For this review, take the finished solid that the model builds, in its own axes (mm). A direction names the side the tool comes from. Give positions to 0.01 mm unless a question says otherwise; leave off trailing zeros. Write each loop counter-clockwise with the first axis right and the second up, starting at its lowest first coordinate (ties: lowest second). Pieces come first, ordered by that corner, then holes. Notation, with made-up numbers: M 40,69 L 68,69 A13 ccw 68,82 Z; hole C 66,55 d5. An arc over 180 degrees is marked long. Use one line per item in the form item = value. Start each with the question number.
Q1. Consider section C-C on z = 25. Write out the cut boundary in (x, y), and give its area (3 significant figures).
Q2. Mouldability with a two-part tool opening along X and no side actions: class faces 3 (the flat face through (25, 202, 50)), 4 (the flat face through (25, 200, 2.5)), 5 (the flat face through (0, 197, 25)) as released by +X, released by -X, zero draft, split by the parting line, or undercut.
Q3. Consider section B-B on x = 18. Write out the cut boundary in (y, z), and give its area (3 significant figures).
Q4. For probe 1 along Z at (x, y) = (38.5, 160); probe 2 along X at (y, z) = (382.5, 3), list the stretches that pass through material, from the lowest coordinate up. Write a range as [from, to].
Q5. Tool access review of faces 1 (the flat face through (25, 0, 1)), 2 (the flat face through (47.5, 200, 25)): name each direction out of +Z, -Z, +X, -X, +Y, -Y from which nothing blocks a thin tool from reaching the whole face with its end or side.
Q6. Consider section A-A on y = 349. Write out the cut boundary in (x, z), and give its area (3 significant figures).
```python
from build123d import *

# Parameters (mm, degrees)
SKETCH1_W           = 50
SKETCH1_H           = 400
BOSS_EXTRUDE1_DEPTH = 50
SKETCH2_W           = 45
SKETCH2_H           = 45
CUT_EXTRUDE1_DEPTH  = 407.201920232
FILLET1_R           = 5
FILLET2_R           = 5


with BuildPart() as part:
    # Sketch1 → Boss-Extrude1 (new body)
    with BuildSketch(Plane.XY):
        with Locations((25, 200)):
            Rectangle(SKETCH1_W, SKETCH1_H)
    extrude(amount=BOSS_EXTRUDE1_DEPTH)

    # Sketch2 → Cut-Extrude1 (cut, through all)
    with BuildSketch(Plane(origin=(0, 400, 0), x_dir=(1, 0, 0), z_dir=(0, 1, 0))):
        with Locations((25, -25)):
            Rectangle(SKETCH2_W, SKETCH2_H)
    extrude(amount=-CUT_EXTRUDE1_DEPTH, mode=Mode.SUBTRACT)

    # Fillet1
    fillet1_edges = [part.edges().sort_by_distance(p)[0] for p in [
        (50, 200, 50),
        (0, 200, 50),
        (50, 200, 0),
        (0, 200, 0),
    ]]
    fillet(fillet1_edges, radius=FILLET1_R)

    # Fillet2
    # the kernel refuses this fillet: 5 mm, written as the material it takes off along each edge
    with BuildSketch(Plane(origin=(47.5, 400, 2.5), x_dir=(0, -1, 0), z_dir=(0, 0, 1)), Plane(origin=(47.5, 400, 47.5), x_dir=(0, -1, 0), z_dir=(-1, 0, 0)), Plane(origin=(2.5, 400, 47.5), x_dir=(0, -1, 0), z_dir=(0, 0, -1)), Plane(origin=(2.5, 400, 2.5), x_dir=(0, -1, 0), z_dir=(1, 0, 0))) as fillet2_piece_1:
        with BuildLine():
            CenterArc((FILLET2_R, FILLET2_R), FILLET2_R, 180, 90)
            Line((0, FILLET2_R), (-FILLET2_R * 0.02, FILLET2_R))
            Line((-FILLET2_R * 0.02, FILLET2_R), (-FILLET2_R * 0.02, -FILLET2_R * 0.02))
            Line((-FILLET2_R * 0.02, -FILLET2_R * 0.02), (FILLET2_R, -FILLET2_R * 0.02))
            Line((FILLET2_R, -FILLET2_R * 0.02), (FILLET2_R, 0))
        make_face()
    extrude(amount=45, mode=Mode.SUBTRACT)
    with BuildSketch(Plane(origin=(47.5, 400, -10), x_dir=(0, -1, 0), z_dir=(0, 0, 1))) as fillet2_piece_2a_section:
        with BuildLine():
            CenterArc((FILLET2_R, FILLET2_R), FILLET2_R, 180, 90)
            Line((0, FILLET2_R), (-FILLET2_R * 0.02, FILLET2_R))
            Line((-FILLET2_R * 0.02, FILLET2_R), (-FILLET2_R * 0.02, -FILLET2_R * 0.02))
            Line((-FILLET2_R * 0.02, -FILLET2_R * 0.02), (FILLET2_R, -FILLET2_R * 0.02))
            Line((FILLET2_R, -FILLET2_R * 0.02), (FILLET2_R, 0))
        make_face()
    fillet2_piece_2a = extrude(amount=57.5, mode=Mode.PRIVATE)
    fillet2_piece_2a = split(fillet2_piece_2a, bisect_by=Plane(origin=(48.631975571, 398.868024429, 2.5), z_dir=(0, 0, -1)), keep=Keep.TOP, mode=Mode.PRIVATE)
    with BuildSketch(Plane(origin=(2.5, 400, 2.5), x_dir=(0, -1, 0), z_dir=(1, 0, 0))) as fillet2_piece_2b_section:
        with BuildLine():
            CenterArc((FILLET2_R, FILLET2_R), FILLET2_R, 180, 90)
            Line((0, FILLET2_R), (-FILLET2_R * 0.02, FILLET2_R))
            Line((-FILLET2_R * 0.02, FILLET2_R), (-FILLET2_R * 0.02, -FILLET2_R * 0.02))
            Line((-FILLET2_R * 0.02, -FILLET2_R * 0.02), (FILLET2_R, -FILLET2_R * 0.02))
            Line((FILLET2_R, -FILLET2_R * 0.02), (FILLET2_R, 0))
        make_face()
    fillet2_piece_2b = extrude(amount=57.5, mode=Mode.PRIVATE)
    fillet2_piece_2b = split(fillet2_piece_2b, bisect_by=Plane(origin=(47.5, 398.868024429, 1.368024429), z_dir=(1, 0, 0)), keep=Keep.TOP, mode=Mode.PRIVATE)
    fillet2_piece_2 = fillet2_piece_2a & fillet2_piece_2b
    add(fillet2_piece_2, mode=Mode.SUBTRACT)
    with BuildSketch(Plane(origin=(60, 400, 47.5), x_dir=(0, -1, 0), z_dir=(-1, 0, 0))) as fillet2_piece_3a_section:
        with BuildLine():
            CenterArc((FILLET2_R, FILLET2_R), FILLET2_R, 180, 90)
            Line((0, FILLET2_R), (-FILLET2_R * 0.02, FILLET2_R))
            Line((-FILLET2_R * 0.02, FILLET2_R), (-FILLET2_R * 0.02, -FILLET2_R * 0.02))
            Line((-FILLET2_R * 0.02, -FILLET2_R * 0.02), (FILLET2_R, -FILLET2_R * 0.02))
            Line((FILLET2_R, -FILLET2_R * 0.02), (FILLET2_R, 0))
        make_face()
    fillet2_piece_3a = extrude(amount=57.5, mode=Mode.PRIVATE)
    fillet2_piece_3a = split(fillet2_piece_3a, bisect_by=Plane(origin=(47.5, 398.868024429, 48.631975571), z_dir=(1, 0, 0)), keep=Keep.TOP, mode=Mode.PRIVATE)
    with BuildSketch(Plane(origin=(47.5, 400, 2.5), x_dir=(0, -1, 0), z_dir=(0, 0, 1))) as fillet2_piece_3b_section:
        with BuildLine():
            CenterArc((FILLET2_R, FILLET2_R), FILLET2_R, 180, 90)
            Line((0, FILLET2_R), (-FILLET2_R * 0.02, FILLET2_R))
            Line((-FILLET2_R * 0.02, FILLET2_R), (-FILLET2_R * 0.02, -FILLET2_R * 0.02))
            Line((-FILLET2_R * 0.02, -FILLET2_R * 0.02), (FILLET2_R, -FILLET2_R * 0.02))
            Line((FILLET2_R, -FILLET2_R * 0.02), (FILLET2_R, 0))
        make_face()
    fillet2_piece_3b = extrude(amount=57.5, mode=Mode.PRIVATE)
    fillet2_piece_3b = split(fillet2_piece_3b, bisect_by=Plane(origin=(48.631975571, 398.868024429, 47.5), z_dir=(0, 0, 1)), keep=Keep.TOP, mode=Mode.PRIVATE)
    fillet2_piece_3 = fillet2_piece_3a & fillet2_piece_3b
    add(fillet2_piece_3, mode=Mode.SUBTRACT)
    with BuildSketch(Plane(origin=(2.5, 400, 60), x_dir=(0, -1, 0), z_dir=(0, 0, -1))) as fillet2_piece_4a_section:
        with BuildLine():
            CenterArc((FILLET2_R, FILLET2_R), FILLET2_R, 180, 90)
            Line((0, FILLET2_R), (-FILLET2_R * 0.02, FILLET2_R))
            Line((-FILLET2_R * 0.02, FILLET2_R), (-FILLET2_R * 0.02, -FILLET2_R * 0.02))
            Line((-FILLET2_R * 0.02, -FILLET2_R * 0.02), (FILLET2_R, -FILLET2_R * 0.02))
            Line((FILLET2_R, -FILLET2_R * 0.02), (FILLET2_R, 0))
        make_face()
    fillet2_piece_4a = extrude(amount=57.5, mode=Mode.PRIVATE)
    fillet2_piece_4a = split(fillet2_piece_4a, bisect_by=Plane(origin=(1.368024429, 398.868024429, 47.5), z_dir=(0, 0, 1)), keep=Keep.TOP, mode=Mode.PRIVATE)
    with BuildSketch(Plane(origin=(47.5, 400, 47.5), x_dir=(0, -1, 0), z_dir=(-1, 0, 0))) as fillet2_piece_4b_section:
        with BuildLine():
            CenterArc((FILLET2_R, FILLET2_R), FILLET2_R, 180, 90)
            Line((0, FILLET2_R), (-FILLET2_R * 0.02, FILLET2_R))
            Line((-FILLET2_R * 0.02, FILLET2_R), (-FILLET2_R * 0.02, -FILLET2_R * 0.02))
            Line((-FILLET2_R * 0.02, -FILLET2_R * 0.02), (FILLET2_R, -FILLET2_R * 0.02))
            Line((FILLET2_R, -FILLET2_R * 0.02), (FILLET2_R, 0))
        make_face()
    fillet2_piece_4b = extrude(amount=57.5, mode=Mode.PRIVATE)
    fillet2_piece_4b = split(fillet2_piece_4b, bisect_by=Plane(origin=(2.5, 398.868024429, 48.631975571), z_dir=(-1, 0, 0)), keep=Keep.TOP, mode=Mode.PRIVATE)
    fillet2_piece_4 = fillet2_piece_4a & fillet2_piece_4b
    add(fillet2_piece_4, mode=Mode.SUBTRACT)
    with BuildSketch(Plane(origin=(2.5, 400, 47.5), x_dir=(0, -1, 0), z_dir=(0, 0, -1))) as fillet2_piece_5a_section:
        with BuildLine():
            CenterArc((FILLET2_R, FILLET2_R), FILLET2_R, 180, 90)
            Line((0, FILLET2_R), (-FILLET2_R * 0.02, FILLET2_R))
            Line((-FILLET2_R * 0.02, FILLET2_R), (-FILLET2_R * 0.02, -FILLET2_R * 0.02))
            Line((-FILLET2_R * 0.02, -FILLET2_R * 0.02), (FILLET2_R, -FILLET2_R * 0.02))
            Line((FILLET2_R, -FILLET2_R * 0.02), (FILLET2_R, 0))
        make_face()
    fillet2_piece_5a = extrude(amount=57.5, mode=Mode.PRIVATE)
    fillet2_piece_5a = split(fillet2_piece_5a, bisect_by=Plane(origin=(1.368024429, 398.868024429, 2.5), z_dir=(0, 0, -1)), keep=Keep.TOP, mode=Mode.PRIVATE)
    with BuildSketch(Plane(origin=(-10, 400, 2.5), x_dir=(0, -1, 0), z_dir=(1, 0, 0))) as fillet2_piece_5b_section:
        with BuildLine():
            CenterArc((FILLET2_R, FILLET2_R), FILLET2_R, 180, 90)
            Line((0, FILLET2_R), (-FILLET2_R * 0.02, FILLET2_R))
            Line((-FILLET2_R * 0.02, FILLET2_R), (-FILLET2_R * 0.02, -FILLET2_R * 0.02))
            Line((-FILLET2_R * 0.02, -FILLET2_R * 0.02), (FILLET2_R, -FILLET2_R * 0.02))
            Line((FILLET2_R, -FILLET2_R * 0.02), (FILLET2_R, 0))
        make_face()
    fillet2_piece_5b = extrude(amount=57.5, mode=Mode.PRIVATE)
    fillet2_piece_5b = split(fillet2_piece_5b, bisect_by=Plane(origin=(2.5, 398.868024429, 1.368024429), z_dir=(-1, 0, 0)), keep=Keep.TOP, mode=Mode.PRIVATE)
    fillet2_piece_5 = fillet2_piece_5a & fillet2_piece_5b
    add(fillet2_piece_5, mode=Mode.SUBTRACT)


solid = part.part
```
Working result:
q1.outline = M 0,0 L 2.5,0 L 2.5,395 A5 ccw 0,399.33 Z; M 47.5,0 L 50,0 L 50,399.33 A5 ccw 47.5,395 Z
q1.area = 1,990 mm²
q2.face_3 = zero draft
q2.face_4 = undercut
q2.face_5 = released by -X
q3.outline = M 0,0 L 399.33,0 A5 ccw 395,2.5 L 0,2.5 Z; M 0,47.5 L 395,47.5 A5 ccw 399.33,50 L 0,50 Z
q3.area = 1,990 mm²
q4.probe_1 = [0, 2.5], [47.5, 50]
q4.probe_2 = [0.42, 2.5], [47.5, 49.58]
q5.face_1 = +Z, -Z, +X, -X, -Y
q5.face_2 = +Y, -Y
q6.outline = M 0,5 A5 ccw 5,0 L 45,0 A5 ccw 50,5 L 50,45 A5 ccw 45,50 L 5,50 A5 ccw 0,45 Z; hole M 2.5,2.5 L 47.5,2.5 L 47.5,47.5 L 2.5,47.5 Z
q6.area = 454 mm²
